The drawing under review shows one solid part. Ordinate dimensions are in mm from its lowest x, y, z. Give positions to 0.01 mm unless a question says otherwise; leave off trailing zeros. Order: outer loops, then holes, each group sorted by start corner. A loop starts at its lowest first (then second) coordinate and runs counter-clockwise, first axis right, second up. Notation, with made-up numbers: (87.5, 7.25) -> (114.5, 7.25) arc R11 cw to (114.5, 15.25) -> close; hole circle Ø11 at (-5.5, 36). An arc over 180 degrees is marked (long way). Return JSON: item names as keys, results as strings. Group by question number.
1) Insertion check: P1, Ø4, axis at y = 15.5, z = 12.5, coming from the -X side. The pin has a flat end and moves straight along its axis. Give the tip position at first contact, or say it passes through.
2) Add section B-B (y = 15). Give the boundary of the cut face in (x, z).
3) Add section A-A (x = 15). Give the boundary of the cut face in (y, z).
4) The part is to be moulded in two halves that separate along Z. For the marked faces 1, 2, 3 and 4, say which applies: released by +Z, released by -Z, zero draft, split by the parting line, or undercut.
5) To check wall thickness, follow line 1 along Z through (x, y) = (15, 8.5); line 2 along X through (y, z) = (12.5, 15.75). State the ranges of each line that lie inside material, in increasing order.
6) Add section C-C (z = 15). Give the boundary of the cut face in (x, y).
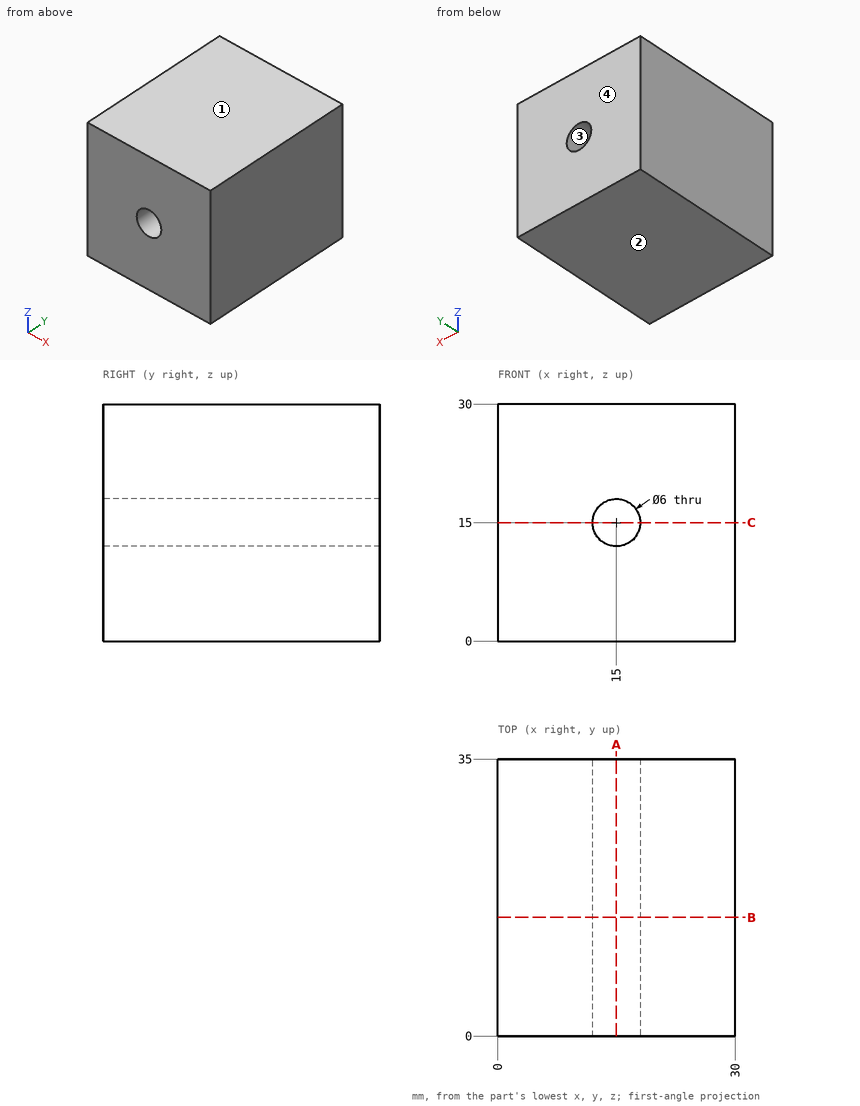
Evaluation:
{
 "1": {"P1": "x = 0"},
 "2": {"outline": "(0, 0) -> (30, 0) -> (30, 30) -> (0, 30) -> close; hole circle Ø6 at (15, 15)"},
 "3": {"outline": "(0, 0) -> (35, 0) -> (35, 12) -> (0, 12) -> close; (0, 18) -> (35, 18) -> (35, 30) -> (0, 30) -> close"},
 "4": {"face 1": "released by +Z", "face 2": "released by -Z", "face 3": "undercut", "face 4": "zero draft"},
 "5": {"line 1": "0 to 12, 18 to 30", "line 2": "0 to 12.1, 17.9 to 30"},
 "6": {"outline": "(0, 0) -> (12, 0) -> (12, 35) -> (0, 35) -> close; (18, 0) -> (30, 0) -> (30, 35) -> (18, 35) -> close"}
}
